Check sheet for the modelled part. Datum: model origin and axes. Units: mm. Give positions to 0.01 mm unless a question says otherwise; leave off trailing zeros. Order: outer loops, then holes, each group sorted by start corner. A loop starts at its lowest first (then second) coordinate and runs counter-clockwise, first axis right, second up. Notation, with made-up numbers: M 44,61.25 L 78,61.25 A20 cw 78,92.25 Z; hole C -16,81 d7. An arc over 180 degrees is marked long. Answer in a Markdown table with one row per item. Add a question column.
from build123d import *

# Parameters (mm, degrees)
BOSS_EXTRUDE1_START = -47.625
SKETCH1_R           = 3.175
SKETCH1_R_2         = 3.2639
BOSS_EXTRUDE1_DEPTH = 6.35


with BuildPart() as part:
    # Sketch1 → Boss-Extrude1 (new body)
    with BuildSketch(Plane(origin=(0, 0, 0), x_dir=(0, 0, -1), z_dir=(1, 0, 0)).offset(BOSS_EXTRUDE1_START)):
        with BuildLine():
            Line((31.75, 95.375), (-84.778478767, 95.375))
            ThreePointArc((-84.778478767, 95.375), (-98.053593602, 96.070719288), (-111.183263501, 98.150254707))
            Line((-111.183263501, 98.150254707), (-128.980358855, 101.933144103))
            ThreePointArc((-128.980358855, 101.933144103), (-136.523496243, 111.080753692), (-129.310151828, 120.490607314))
            Line((-129.310151828, 120.490607314), (-27.710151828, 145.890607314))
            ThreePointArc((-27.710151828, 145.890607314), (-26.563795587, 146.103634477), (-25.4, 146.175))
            Line((-25.4, 146.175), (0, 146.175))
            ThreePointArc((0, 146.175), (3.645059693, 145.449952547), (6.735192091, 143.385192091))
            Line((6.735192091, 143.385192091), (38.485192091, 111.635192091))
            ThreePointArc((38.485192091, 111.635192091), (40.549952547, 101.254940307), (31.75, 95.375))
        make_face()
        with Locations((-127, 111.25)):
            Circle(SKETCH1_R, mode=Mode.SUBTRACT)
        with Locations((-53.558195394, 129.610451151)):
            Circle(SKETCH1_R_2, mode=Mode.SUBTRACT)
        with Locations((0, 136.65)):
            Circle(SKETCH1_R, mode=Mode.SUBTRACT)
        with Locations((-31.75, 104.9)):
            Circle(SKETCH1_R, mode=Mode.SUBTRACT)
        with Locations((0, 104.9)):
            Circle(SKETCH1_R, mode=Mode.SUBTRACT)
        with Locations((31.75, 104.9)):
            Circle(SKETCH1_R, mode=Mode.SUBTRACT)
        with Locations((-25.4, 136.65)):
            Circle(SKETCH1_R, mode=Mode.SUBTRACT)
    extrude(amount=-BOSS_EXTRUDE1_DEPTH)


solid = part.part
Q1. Go/stop test with flat-tipped pins: pin 1 (1.5 mm diameter, centred on x = -52.5, z = 105.5, fed in from -Y); pin 2 (2 mm diameter, centred on x = -53, y = 114.5, fed in from -Z). Record where each tip stops, or that it passes through.
Q2. Cross-section at A-A (z = 126). Record the boundary of the cut face in (x, y) (3 decimals), and give its area (3 significant figures).
Q3. Thickness scan on probe 1 along Y at (x, z) = (-50.25, 25.4) (3 decimals); probe 2 along Y at (x, z) = (-51, -31.75) (3 decimals); probe 3 along Y at (x, z) = (-52.25, 35.5) (3 decimals). Record the ranges inside material, lowest first.
Q4. Cross-section at D-D (y = 104.9). Record the boundary of the cut face in (x, z) (3 decimals), and give its area (3 significant figures).
Q5. Cross-section at C-C (y = 136.65). Record the boundary of the cut face in (x, z) (3 decimals).
Q6. Cross-section at B-B (x = -48.75). Record the boundary of the cut face in (y, z) (3 decimals).
Q7. Draft check along Y on faces 1 (the flat face through (-50.76, 127.73, -22.39)), 2 (the flat face through (-47.625, 115, 46)), 3 (the cylindrical face through (-50.756, 126.424, 54.266)). Enter one of: pulls with the +Y half, pulls with the -Y half, needs draft (parallel to the pull), parting line crosses it, or undercut.
Values follow:
| question | item | result |
|---|---|---|
| 1 | pin 1 | y = 96.96 |
| 1 | pin 2 | z = -36.62 |
| 2 | outline | M -53.975,101.3 L -47.625,101.3 L -47.625,108.237 L -53.975,108.237 Z; M -53.975,114.263 L -47.625,114.263 L -47.625,121.318 L -53.975,121.318 Z |
| 2 | area | 88.8 mm² |
| 3 | probe 1 | 95.375 to 133.475, 139.825 to 146.175 |
| 3 | probe 2 | 95.375 to 101.725, 108.075 to 118.37 |
| 3 | probe 3 | 95.375 to 143.943 |
| 4 | outline | M -53.975,-41.275 L -47.625,-41.275 L -47.625,-34.925 L -53.975,-34.925 Z; M -53.975,-28.575 L -47.625,-28.575 L -47.625,-3.175 L -53.975,-3.175 Z; M -53.975,3.175 L -47.625,3.175 L -47.625,28.575 L -53.975,28.575 Z; M -53.975,34.925 L -47.625,34.925 L -47.625,134.1 L -53.975,134.1 Z |
| 4 | area | 993 mm² |
| 5 | outline | M -53.975,-13.47 L -47.625,-13.47 L -47.625,-3.175 L -53.975,-3.175 Z; M -53.975,3.175 L -47.625,3.175 L -47.625,22.225 L -53.975,22.225 Z; M -53.975,28.575 L -47.625,28.575 L -47.625,64.673 L -53.975,64.673 Z |
| 6 | outline | M 95.375,-31.75 A9.525 ccw 111.635,-38.485 L 143.385,-6.735 A9.525 ccw 146.175,0 L 146.175,25.4 A9.525 ccw 145.891,27.71 L 120.491,129.31 A9.525 ccw 101.933,128.98 L 98.15,111.183 A127 ccw 95.375,84.778 Z; hole C 104.9,-31.75 d6.35; hole C 104.9,0 d6.35; hole C 104.9,31.75 d6.35; hole C 111.25,127 d6.35; hole C 129.61,53.558 d6.528; hole C 136.65,0 d6.35; hole C 136.65,25.4 d6.35 |
| 7 | face 1 | pulls with the +Y half |
| 7 | face 2 | needs draft |
| 7 | face 3 | undercut |
